Build history of the part. All positions in model axes, mm. Face numbers are marked on the shaded views. A direction names the side the tool comes from. Coordinates: 2 decimals unless noted, no trailing zeros. Write each loop counter-clockwise with the first axis right and the second up, starting at its lowest first coordinate (ties: lowest second). Pieces come first, ordered by that corner, then holes.
Autodesk Inventor part; units mm, degrees
ref_plane "YZ Plane" through (0, 0, 0) normal (1, 0, 0) x (0, 1, 0)
ref_plane "XZ Plane" through (0, 0, 0) normal (0, 1, 0) x (-1, 0, 0)
ref_plane "XY Plane" through (0, 0, 0) normal (0, 0, 1) x (1, 0, 0)
sketch "Sketch1" plane through (0, 0, 0) normal (0, 1, 0) x (-1, 0, 0)
  line L0 (18, 30) -> (-18, 30)
  line L1 (-18, 30) -> (-18, -30)
  line L2 (-18, -30) -> (18, -30)
  line L3 (18, -30) -> (18, 30)
  line L4 (18, 30) -> (-18, -30) construction
  line L5 (-18, 30) -> (18, -30) construction
  circle A0 centre (9, 20) radius 3
  circle A1 centre (9, 5) radius 3
  circle A2 centre (-9, 18) radius 3
  circle A3 centre (-9, 6) radius 3
  circle A4 centre (-9, -6) radius 3
  circle A5 centre (-9, -18) radius 3
  circle A6 centre (9, -10) radius 3
  circle A7 centre (9, -20) radius 1.5
  line L6 (21, 33) -> (-21, 33)
  line L7 (-21, 33) -> (-21, -33)
  line L8 (-21, -33) -> (21, -33)
  line L9 (21, -33) -> (21, 33)
  line L10 (21, 33) -> (-21, -33) construction
  line L11 (-21, 33) -> (21, -33) construction
  point P0 (0, 0)
  dimension "d0" = 36
  dimension "d1" = 60
  dimension "d2" = 6
  dimension "d3" = 6
  dimension "d4" = 6
  dimension "d5" = 6
  dimension "d6" = 6
  dimension "d7" = 6
  dimension "d8" = 6
  dimension "d9" = 3
  dimension "d10" = 10
  dimension "d11" = 5
  dimension "d12" = 9
  dimension "d13" = 9
  dimension "d14" = 9
  dimension "d15" = 9
  dimension "d16" = 10
  dimension "d17" = 10
  dimension "d18" = 9
  dimension "d19" = 9
  dimension "d20" = 9
  dimension "d21" = 9
  dimension "d22" = 12
  dimension "d23" = 12
  dimension "d24" = 12
  dimension "d25" = 12
  dimension "d26" = 3
  dimension "d27" = 3
extrude "Extrusion1" add sketch "Sketch1" along normal blind 3 contours L3 L2 L1 L0 | L9 L8 L7 L6
sketch "Sketch2" plane through (0, 0, 0) normal (0, -1, 0) x (1, 0, 0)
  line L0 (18, 30) -> (-18, 30)
  line L1 (-18, 30) -> (-18, -30)
  line L2 (-18, -30) -> (18, -30)
  line L3 (18, -30) -> (18, 30)
  line L4 (18, 30) -> (-18, -30) construction
  line L5 (-18, 30) -> (18, -30) construction
  line L6 (16, 28) -> (-16, 28)
  line L7 (-16, 28) -> (-16, -28)
  line L8 (-16, -28) -> (16, -28)
  line L9 (16, -28) -> (16, 28)
  line L10 (16, 28) -> (-16, -28) construction
  line L11 (-16, 28) -> (16, -28) construction
  point P0 (0, 0)
  dimension "d30" = 36
  dimension "d31" = 60
  dimension "d32" = 2
  dimension "d33" = 2
extrude "Extrusion2" add sketch "Sketch2" along normal blind 10
fillet "Fillet1" radius 2 8 edges at (21, 3, 0) (0, 3, -33) (0, 3, 33) (-21, 3, 0) (21, 1.5, 33) (21, 1.5, -33) (-21, 1.5, -33) (-21, 1.5, 33)
fillet "Fillet2" radius 2 8 edges at (-16, -5, -28) (0, 0, -28) (16, -5, -28) (16, 0, 0) (16, -5, 28) (0, 0, 28) (-16, -5, 28) (-16, 0, 0)
properties part number "vstup"
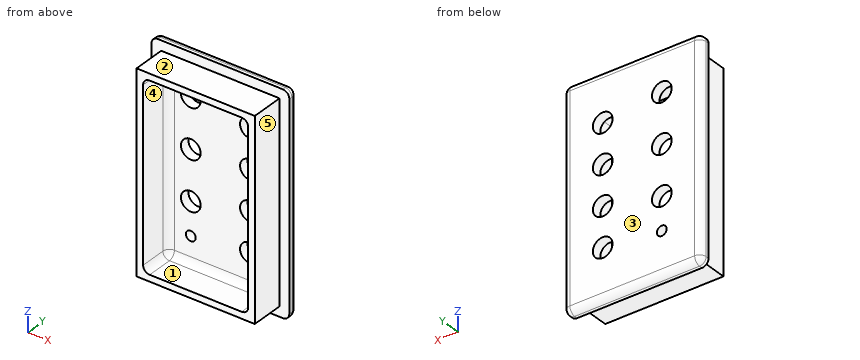
1. Probe line 1 along Z through (x, y) = (-9, 0.75); line 2 along X through (y, z) = (-8.75, -25.5); line 3 along Z through (x, y) = (-4.5, -2.25). List the from-to ranges inside material, lowest first.
Computed values:
line 1: z = -33 to -21.5, -18.5 to -13, -7 to 2, 8 to 17, 23 to 33
line 2: x = -18 to -16, 16 to 18
line 3: z = -30 to -28, 28 to 30
2. Mould opens along X. For the marked faces 3, 4 and 5 say: +X half, -X half, draft (parallel to the pull), parting line (faces both ways), or undercut.
Computed values:
face 3: draft
face 4: undercut
face 5: +X half
3. Saw through at A-A on z = -10. List the corners of the cut face in (x, y), plus the area to 3 significant figures.
Computed values:
outline: (-21, 0) - (-18, 0) - (-18, -10) - (-16, -10) - (-16, -2) arc R2 cw to (-14, 0) - (-12, 0) - (-12, 3) - (-19, 3) arc R2 ccw to (-21, 1) - close; (-6, 0) - (14, 0) arc R2 cw to (16, -2) - (16, -10) - (18, -10) - (18, 0) - (21, 0) - (21, 1) arc R2 ccw to (19, 3) - (-6, 3) - close
area: 148 mm2
4. Saw through at B-B on x = -9. State how many separate pieces and enclosed holes the cut face has, plus the area to 3 significant figures.
Computed values:
separate pieces: 5
enclosed holes: 0
area: 175 mm2
5. 3-axis set-ups, long thin cutter, end or side, ignore diameter. For the marked faces 1 and 2: which of +Z, -Z, +X, -X, +Y, -Y reach the whole face in a straight line?
Computed values:
face 1: -Y
face 2: +Z, +X, -X, -Y
6. Saw through at C-C on y = -3.25. List the corners of the cut face in (x, z), plus the area to 3 significant figures.
Computed values:
outline: (-18, -30) - (18, -30) - (18, 30) - (-18, 30) - close; hole (-16, -26) arc R2 ccw to (-14, -28) - (14, -28) arc R2 ccw to (16, -26) - (16, 26) arc R2 ccw to (14, 28) - (-14, 28) arc R2 ccw to (-16, 26) - close
area: 371 mm2
7. Saw through at D-D on z = 5. List the corners of the cut face in (x, y).
Computed values:
outline: (-21, 0) - (-18, 0) - (-18, -10) - (-16, -10) - (-16, -2) arc R2 cw to (-14, 0) - (-12, 0) - (-12, 3) - (-19, 3) arc R2 ccw to (-21, 1) - close; (-6, 0) - (6.17, 0) - (6.17, 3) - (-6, 3) - close; (11.83, 0) - (14, 0) arc R2 cw to (16, -2) - (16, -10) - (18, -10) - (18, 0) - (21, 0) - (21, 1) arc R2 ccw to (19, 3) - (11.83, 3) - close
8. Flat gauge pins, fed straight in: pin 1 (1 mm diameter, centred on x = 2, y = -3.5, fed in from -Z); pin 2 (5.5 mm diameter, centred on x = -9, z = -10, fed in from +Y); pin 3 (4 mm diameter, centred on y = -5, z = -11, fed in from +X); pin 4 (2 mm diameter, centred on x = -6, y = -0.5, fed in from +Z). Where does each tip first touch, or does it go through?
Computed values:
pin 1: stops at z = -30
pin 2: passes through
pin 3: stops at x = 18
pin 4: stops at z = 33
